```python
from build123d import *

# Parameters (mm, degrees)
CROQUIS1_R              = 8
SALIENTE_EXTRUIR1_DEPTH = 7
CROQUIS2_R              = 6.1
SALIENTE_EXTRUIR2_DEPTH = 9.8
CROQUIS3_R              = 8
SALIENTE_EXTRUIR3_DEPTH = 1.2
CROQUIS4_R              = 2.5
CORTAR_EXTRUIR1_DEPTH   = 22.260291625
CHAFL_N1_SIZE           = 0.5
CROQUIS5_R              = 1.5
CORTAR_EXTRUIR2_DEPTH   = 22.260291625
CROQUIS6_R              = 1.5
CORTAR_EXTRUIR3_DEPTH   = 22.260291701


with BuildPart() as part:
    # Croquis1 → Saliente-Extruir1 (new body)
    with BuildSketch(Plane.XY):
        Circle(CROQUIS1_R)
    extrude(amount=SALIENTE_EXTRUIR1_DEPTH)

    # Croquis2 → Saliente-Extruir2 (add)
    with BuildSketch(Plane.XY.offset(7)):
        Circle(CROQUIS2_R)
    extrude(amount=SALIENTE_EXTRUIR2_DEPTH)

    # Croquis3 → Saliente-Extruir3 (add)
    with BuildSketch(Plane.XY.offset(16.8)):
        Circle(CROQUIS3_R)
    extrude(amount=SALIENTE_EXTRUIR3_DEPTH)

    # Croquis4 → Cortar-Extruir1 (cut, through all)
    with BuildSketch(Plane.XY.offset(18)):
        Circle(CROQUIS4_R)
    extrude(amount=-CORTAR_EXTRUIR1_DEPTH, mode=Mode.SUBTRACT)

    # Chaflán1
    chafl_n1_edges = [part.edges().sort_by_distance(p)[0] for p in [
        (-2.5, 0, 0),
        (-2.5, 0, 18),
        (-8, 0, 0),
    ]]
    chamfer(chafl_n1_edges, length=CHAFL_N1_SIZE)

    # Croquis5 → Cortar-Extruir2 (cut, through all)
    with BuildSketch(Plane(origin=(0, 0, 0), x_dir=(0, 0, -1), z_dir=(1, 0, 0))):
        with Locations((-3.5, 0)):
            Circle(CROQUIS5_R)
    extrude(amount=-CORTAR_EXTRUIR2_DEPTH, mode=Mode.SUBTRACT)

    # Croquis6 → Cortar-Extruir3 (cut, through all)
    with BuildSketch(Plane(origin=(0, 0, 0), x_dir=(1, 0, 0), z_dir=(0, 1, 0))):
        with Locations(Location((0, -3.5, 0), (0, 0, 270))):
            Circle(CROQUIS6_R)
    extrude(amount=-CORTAR_EXTRUIR3_DEPTH, mode=Mode.SUBTRACT)


solid = part.part
```
Here's how the part is built. I have some questions about the finished solid (model axes, mm). A direction names the side the tool comes from. Round coordinates to 2 decimals unless told otherwise and drop trailing zeros. Order: outer loops, then holes, each group sorted by start corner. A loop starts at its lowest first (then second) coordinate and runs counter-clockwise, first axis right, second up. Notation, with made-up numbers: M 74.5,75.25 L 131.5,75.25 A18 ccw 131.5,80.25 Z; hole C 23,-13 d1. An arc over 180 degrees is marked long. One line per question, with ' | ' between items.
1) For faces 1 (the face through (-1.73, -7.81, 17.39)), 2 (the face through (-4.958, 1.487, 3.695)), 3 (the face through (-2, -6, 16.8)), which set-ups out of +Z, -Z, +X, -X, +Y, -Y let a thin tool reach every point of the face, with its end or its side?
Working result:
face 1: +Z, -Z | face 2: -X | face 3: none
2) I need wall thicknesses on line 1 along Y through (x, z) = (0, 10.75); line 2 along X through (y, z) = (0, 6.5); line 3 along Z through (x, y) = (-1.75, 6.5). Which ranges of each line are inside material? Lowest first, please.
Working result:
line 1: -6.1 to -2.5, 2.5 to 6.1 | line 2: -8 to -2.5, 2.5 to 8 | line 3: 0 to 7, 16.8 to 18
3) I want a section at A-A, the plane y = 0. Write out the boundary of the cut face in (x, z).
Working result:
outline: M -8,0.5 L -7.5,0 L -3,0 L -2.5,0.5 L -2.5,2 L -8,2 Z; M -8,5 L -2.5,5 L -2.5,17.5 L -3,18 L -8,18 L -8,16.8 L -6.1,16.8 L -6.1,7 L -8,7 Z; M 2.5,0.5 L 3,0 L 7.5,0 L 8,0.5 L 8,7 L 6.1,7 L 6.1,16.8 L 8,16.8 L 8,18 L 3,18 L 2.5,17.5 Z
4) If we mould it in two halves opening along X, with no side actions, what happens to faces 4 (the face through (-6.094, 0.268, 11.831)), 5 (the face through (1.487, -4.96, 3.305)), 6 (the face through (-2, -6, 7))? For each: +X half, -X half, draft (parallel to the pull), parting line (faces both ways), or undercut.
Working result:
face 4: parting line | face 5: undercut | face 6: draft
5) I want a section at D-D, the plane z = 14.5. Write out the boundary of the cut face in (x, y), then the cut area to 3 significant figures.
Working result:
outline: C 0,0 d12.2; hole C 0,0 d5 | area: 97.3 mm²
6) I want a section at C-C, the plane z = 3.5. Write out the boundary of the cut face in (x, y).
Working result:
outline: M -7.86,-1.5 A8 ccw -1.5,-7.86 L -1.5,-2 A2.5 cw -2,-1.5 Z; M -7.86,1.5 L -2,1.5 A2.5 cw long 1.5,-2 L 1.5,-7.86 A8 ccw long Z
7) For pin 1 Ø1.5 at (y, z) = (6, 6) entering from -X; pin 2 Ø5 at (x, z) = (2.5, 15) entering from +Y; pin 3 Ø2 at (x, z) = (5, 14) entering from -Y, each with a flat end and sliding along its axis, tell me the tip position at first contact or that it passes through.
Working result:
pin 1: x = -6.04 | pin 2: y = 7.96 | pin 3: y = -4.61
